The model under review builds one solid part; all positions refer to its coordinate system, in mm. A direction names the side the tool comes from. Round coordinates to 2 decimals unless told otherwise and drop trailing zeros. Order: outer loops, then holes, each group sorted by start corner. A loop starts at its lowest first (then second) coordinate and runs counter-clockwise, first axis right, second up. Notation, with made-up numbers: M 65.5,36.25 L 122.5,36.25 A36 cw 122.5,73.25 Z; hole C 54.5,-22 d5. An arc over 180 degrees is marked long. Answer as a JSON object with one key per item and string values. Group by question number.
1. Clearance check with flat-ended pins moving along their axes: P1, Ø4.5, axis at x = 4.5, z = 50, coming from the -Y side; P2, Ø4.5, axis at x = 4.5, z = 130, coming from the +Y side. State where each tip first meets the part, or that it passes through.
2. Mouldability with a two-part tool opening along Z and no side actions: class faces 1 (the face through (9, 2, 69)), 2 (the face through (3.47, 1.22, 48.65)), 3 (the face through (5, 3, 140)) as released by +Z, released by -Z, zero draft, split by the parting line, or undercut.
3. Add section B-B on z = 9.5. State the section outline as (x, y) points, and give its area (3 significant figures).
4. Machinability: for faces 4 (the face through (5.371, 4.428, 32.766)), 5 (the face through (2.84, 1.22, 9.63)), which of the approach directions +Z, -Z, +X, -X, +Y, -Y give a long, thin tool a straight path to every point of the face, cutting with its end or side? Answer none if there is none.
5. Add section A-A on z = 30. State the section outline as (x, y) points, and give its area (3 significant figures).
6. To check wall thickness, follow probe 1 along X at (y, z) = (1.7, 50); probe 2 along Y at (x, z) = (8.75, 68); probe 3 along X at (y, z) = (4, 131.5). State the ranges of each line that lie inside material, in increasing order. Write a range as [from, to].
```python
from build123d import *

# Parameters (mm, degrees)
BOSS_EXTRUDE1_DEPTH = 140
SKETCH2_R           = 2.9
CUT_EXTRUDE1_DEPTH  = 4
SKETCH3_R           = 1.7
CUT_EXTRUDE2_DEPTH  = 141.346001012


with BuildPart() as part:
    # Sketch1 → Boss-Extrude1 (new body)
    with BuildSketch(Plane.XY):
        Polygon((9, 6.4), (9, 4.9), (8.2, 4.45), (9, 4), (9, 0), (0, 0), (0, 4), (0.8, 4.45), (0, 4.9), (0, 6.4), align=None)
    extrude(amount=BOSS_EXTRUDE1_DEPTH)

    # Sketch2 → Cut-Extrude1 (cut)
    with BuildSketch(Plane(origin=(0, 6.4, 0), x_dir=(1, 0, 0), z_dir=(0, 1, 0))):
        with Locations(Location((4.5, -130, 0), (0, 0, 270))):
            Circle(SKETCH2_R)
        with Locations(Location((4.5, -110, 0), (0, 0, 270))):
            Circle(SKETCH2_R)
        with Locations(Location((4.5, -90, 0), (0, 0, 270))):
            Circle(SKETCH2_R)
        with Locations(Location((4.5, -70, 0), (0, 0, 270))):
            Circle(SKETCH2_R)
        with Locations(Location((4.5, -50, 0), (0, 0, 270))):
            Circle(SKETCH2_R)
        with Locations(Location((4.5, -30, 0), (0, 0, 270))):
            Circle(SKETCH2_R)
        with Locations(Location((4.5, -10, 0), (0, 0, 270))):
            Circle(SKETCH2_R)
    extrude(amount=-CUT_EXTRUDE1_DEPTH, mode=Mode.SUBTRACT)

    # Sketch3 → Cut-Extrude2 (cut, through all)
    with BuildSketch(Plane(origin=(0, 2.4, 0), x_dir=(1, 0, 0), z_dir=(0, 1, 0))):
        with Locations(Location((4.5, -130, 0), (0, 0, 270))):
            Circle(SKETCH3_R)
        with Locations(Location((4.5, -110, 0), (0, 0, 270))):
            Circle(SKETCH3_R)
        with Locations(Location((4.5, -90, 0), (0, 0, 270))):
            Circle(SKETCH3_R)
        with Locations(Location((4.5, -70, 0), (0, 0, 270))):
            Circle(SKETCH3_R)
        with Locations(Location((4.5, -50, 0), (0, 0, 270))):
            Circle(SKETCH3_R)
        with Locations(Location((4.5, -30, 0), (0, 0, 270))):
            Circle(SKETCH3_R)
        with Locations(Location((4.5, -10, 0), (0, 0, 270))):
            Circle(SKETCH3_R)
    extrude(amount=-CUT_EXTRUDE2_DEPTH, mode=Mode.SUBTRACT)


solid = part.part
```
Recorded:
{
 "1": {"P1": "stops at y = 0", "P2": "stops at y = 2.4"},
 "2": {"face 1": "zero draft", "face 2": "undercut", "face 3": "released by +Z"},
 "3": {"outline": "M 0,0 L 2.88,0 L 2.88,2.4 L 1.64,2.4 L 1.64,6.4 L 0,6.4 L 0,4.9 L 0.8,4.45 L 0,4 Z; M 6.12,0 L 9,0 L 9,4 L 8.2,4.45 L 9,4.9 L 9,6.4 L 7.36,6.4 L 7.36,2.4 L 6.12,2.4 Z", "area": "26.2 mm²"},
 "4": {"face 4": "+Y", "face 5": "+Y, -Y"},
 "5": {"outline": "M 0,0 L 2.8,0 L 2.8,2.4 L 1.6,2.4 L 1.6,6.4 L 0,6.4 L 0,4.9 L 0.8,4.45 L 0,4 Z; M 6.2,0 L 9,0 L 9,4 L 8.2,4.45 L 9,4.9 L 9,6.4 L 7.4,6.4 L 7.4,2.4 L 6.2,2.4 Z", "area": "25.5 mm²"},
 "6": {"probe 1": "x = [0, 2.8], [6.2, 9]", "probe 2": "y = [0, 4.14], [4.76, 6.4]", "probe 3": "x = [0, 2.02], [6.98, 9]"}
}
